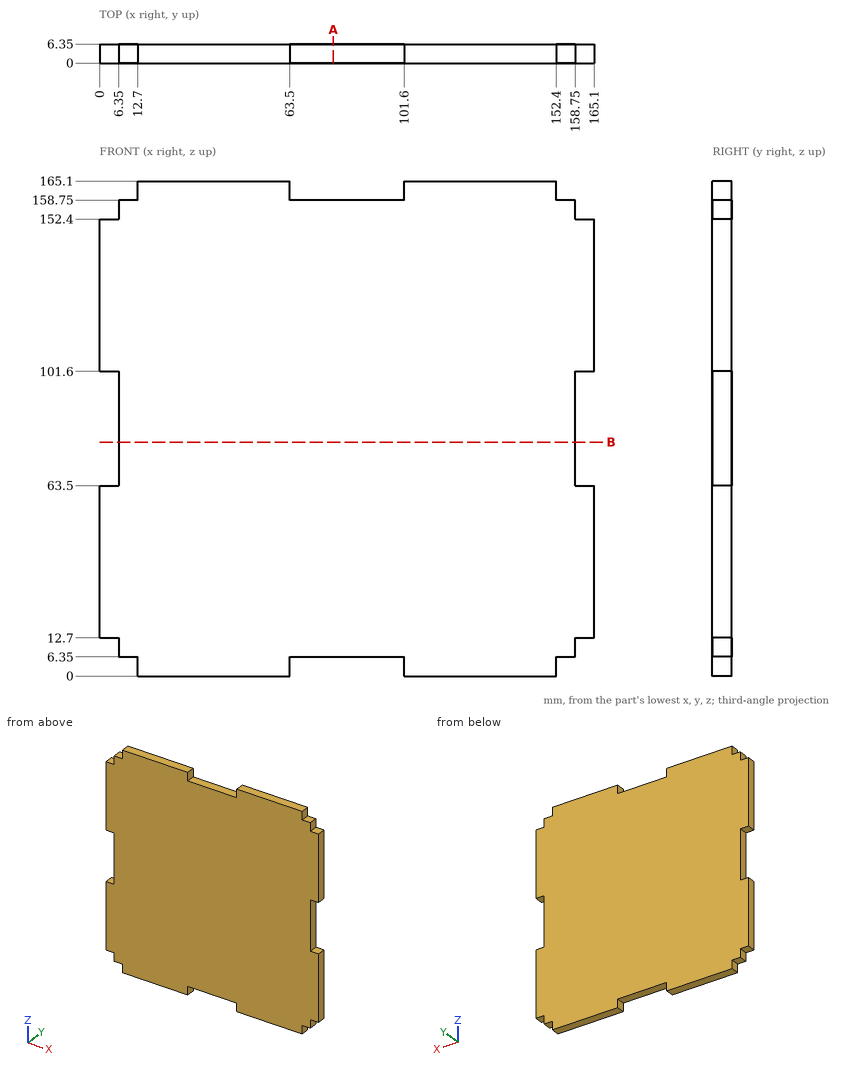
Drawing for the job (mm, zero at the part's lowest x, y, z). Round coordinates to 2 decimals unless told otherwise and drop trailing zeros. Loops run counter-clockwise (first coordinate to the right, second up) from the corner with the lowest first, then second, coordinate; pieces in that order, holes last.
1. Band-saw the part on A-A, the plane x = 78. List the corners of the cut face in (y, z), and give its area (3 significant figures).
Check values:
outline: (0, 6.35) - (6.35, 6.35) - (6.35, 158.75) - (0, 158.75) - close
area: 968 mm2
2. Wall check: probe 1 along X at (y, z) = (2.25, 87). Give the ranges that are in metal, low to high.
Check values:
probe 1: x = 6.35 to 158.75
3. Band-saw the part on B-B, the plane z = 78. List the corners of the cut face in (x, y), and give its area (3 significant figures).
Check values:
outline: (6.35, 0) - (158.75, 0) - (158.75, 6.35) - (6.35, 6.35) - close
area: 968 mm2
4. Drop flat-ended pins along their axis: P1, Ø1, axis at y = 2.5, z = 65.5, coming from the -X side; P2, Ø1.9, axis at y = 4, z = 4, coming from the +X side; P3, Ø1.9, axis at x = 9.5, y = 4.5, coming from the -Z side. Give the stop position or say it passes through.
Check values:
P1: stops at x = 6.35
P2: stops at x = 152.4
P3: stops at z = 6.35
